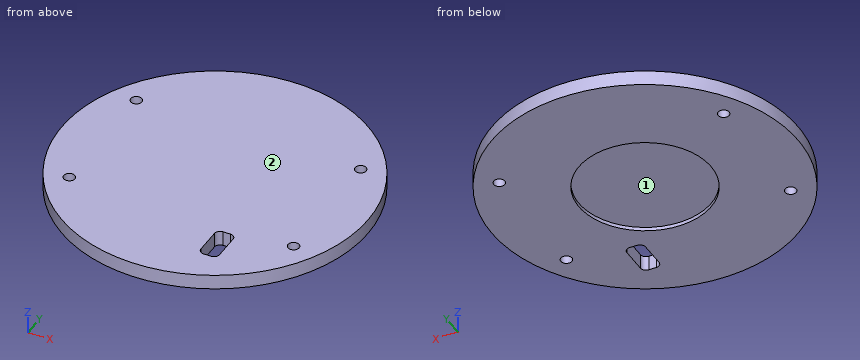
Autodesk Inventor part; units mm, degrees
ref_plane "Work Plane3" through (0, 0, 0) normal (0, 0, 1) x (1, 0, 0)
ref_plane "Work Plane4" through (0, 0, 0) normal (0, 0, 1) x (1, 0, 0)
ref_plane "YZ Plane" through (0, 0, 0) normal (1, 0, 0) x (0, 1, 0)
sketch "Sketch1" plane through (0, 0, 0) normal (0, 0, 1) x (1, 0, 0)
  circle A0 centre (0, 0) radius 41
  circle A1 centre (0, 0) radius 17.705
  circle A2 centre (0, 0) radius 15
  circle A3 centre (0, 15) radius 0.75
  circle A4 centre (-10.6066, 10.6066) radius 0.75
  circle A5 centre (-15, 0) radius 0.75
  circle A6 centre (-10.6066, -10.6066) radius 0.75
  circle A7 centre (0, -15) radius 0.75
  circle A8 centre (10.6066, -10.6066) radius 0.75
  circle A9 centre (15, 0) radius 0.75
  circle A10 centre (10.6066, 10.6066) radius 0.75
  dimension "d4" = 30
  dimension "d0" = 82
  dimension "d3" = 35.41
  dimension "d5" = 1.5
  dimension "d6" = 360
sketch "Sketch2" plane through (0, 0, 0) normal (0, 0, 1) x (1, 0, 0)
  circle A0 centre (-30.094, -17.375) radius 1.5
  circle A1 centre (-30.094, 17.375) radius 1.5
  circle A2 centre (30.094, 17.375) radius 1.5
  circle A3 centre (30.094, -17.375) radius 1.5
  point P0 (0, 0)
  dimension "d7" = 3
  dimension "d8" = 3
  dimension "d9" = 3
  dimension "d10" = 3
  dimension "d11" = 17.375
  dimension "d12" = 30.094
  dimension "d13" = 30.094
  dimension "d14" = 17.375
  dimension "d15" = 17.375
  dimension "d16" = 30.094
  dimension "d17" = 17.375
  dimension "d18" = 30.094
extrude "Extrusion1" add sketch "Sketch1" against normal blind 4 contours A0 | A1 | A2 A9 | A2 A9 | A9 A2 A8 A7 A6 A5 A4 A3 A10 | A10 A2 | A2 A10 | A8 A2 | A2 A8 | A3 A2 | A2 A3 | A7 A2 | A2 A7 | A4 A2 | A2 A4 | A6 A2 | A2 A6 | A5 A2 | A2 A5
extrude "Extrusion2" cut sketch "Sketch2" against normal blind 4
ref_plane "Work Plane1" through (0, 0, -4) normal (0, 0, 1) x (1, 0, 0)
ref_plane "Work Plane2" through (0, 0, -4) normal (0, 0, 1) x (1, 0, 0)
ref_plane "Work Plane3" through (0, 0, 0) normal (0, 0, 1) x (1, 0, 0)
sketch "Sketch5" plane through (0, 0, 0) normal (0, 0, 1) x (1, 0, 0)
  line L0 (11, -30) -> (16, -30)
  line L1 (16, -30) -> (16, -20)
  line L2 (16, -20) -> (11, -20)
  line L3 (11, -20) -> (11, -30)
  point P0 (0, 0)
  point P1 (13.5, -20)
  point P2 (13.5, -30)
  point P3 (16, -25)
  dimension "d44" = 5
  dimension "d45" = 10
  dimension "d54" = 11
  dimension "d55" = 20
extrude "Extrusion5" cut sketch "Sketch5" against normal blind 4
fillet "Fillet1" radius 1.5 4 edges at (11, -20, -2) (11, -30, -2) (16, -20, -2) (16, -30, -2)
ref_plane "Work Plane4" through (0, 0, 0) normal (0, 0, 1) x (1, 0, 0)
ref_plane "Work Plane5" through (0, 0, -4) normal (0, 0, -1) x (-1, 0, 0)
sketch "Sketch7" plane through (0, 0, -4) normal (0, 0, -1) x (-1, 0, 0)
  circle A0 centre (0, 0) radius 17.705
  circle A1 centre (0, 0) radius 15
  circle A2 centre (0, 15) radius 2.5
  circle A3 centre (-10.6066, 10.6066) radius 2.5
  circle A4 centre (-15, 0) radius 2.5
  circle A5 centre (-10.6066, -10.6066) radius 2.5
  circle A6 centre (0, -15) radius 2.5
  circle A7 centre (10.6066, -10.6066) radius 2.5
  circle A8 centre (15, 0) radius 2.5
  circle A9 centre (10.6066, 10.6066) radius 2.5
  circle A10 centre (0, 0) radius 4.25
  circle A11 centre (0, 0) radius 2.5
  point P0 (0, 0)
  point P1 (0, 0)
  point P2 (0, -4)
  point P3 (0, -19)
  dimension "d60" = 35.41
  dimension "d61" = 5
  dimension "d62" = 360
  dimension "d63" = 8.5
  dimension "d64" = 5
  dimension "d65" = 15
  dimension "d66" = 15
extrude "Extrusion6" cut sketch "Sketch7" against normal blind 1 contours A0 | A1 A8 | A1 A8 | A8 A1 A7 A6 A5 A4 A3 A2 A9 | A9 A1 | A1 A9 | A7 A1 | A1 A7 | A2 A1 | A1 A2 | A6 A1 | A1 A6 | A3 A1 | A1 A3 | A5 A1 | A1 A5 | A4 A1 | A1 A4 | A10 | A11
properties part number "lower-plate_3DPrint"
Part model, mm, in its own coordinate system. Face numbers are marked on the shaded views. Give positions to 0.01 mm unless a question says otherwise; leave off trailing zeros. Write each loop counter-clockwise with the first axis right and the second up, starting at its lowest first coordinate (ties: lowest second). Pieces come first, ordered by that corner, then holes. Notation, with made-up numbers: M 21.25,17.5 L 39.25,17.5 A6 ccw 39.25,21.5 Z; hole C -29,-23 d11. An arc over 180 degrees is marked long. Use CSV: the item, a comma, the result in double quotes.
Item 1: Pull direction X, two halves, no side cores. Call the marked faces 1 and 2: +X half, -X half, draft (parallel to the pull), parting line (faces both ways), or undercut.
Taken from the geometry:
face 1,"undercut"
face 2,"draft"
Item 2: Pin check, flat tips, straight feed: P1, Ø3.5, axis at x = 30.094, y = -17.375, coming from the +Z side; P2, Ø1, axis at x = 14, z = -2, coming from the +Y side; P3, Ø1, axis at y = -10, z = -1.5, coming from the +X side; P4, Ø2, axis at y = -24, z = -1.5, coming from the +X side. Stop position of each tip, or through.
Taken from the geometry:
P1,"stops at z = 0"
P2,"stops at y = 38.71"
P3,"stops at x = 39.88"
P4,"stops at x = 33.94"
Item 3: Drill centre lines: probe 1 along Y at (x, z) = (0, -3.65) (3 decimals); probe 2 along Y at (x, z) = (-31, -3); probe 3 along Y at (x, z) = (-16, -3.6). Where is each one in solid material? Low to high.
Taken from the geometry:
probe 1,"y = -41 to -17.705, 17.705 to 41"
probe 2,"y = -26.83 to -18.57, -16.18 to 16.18, 18.57 to 26.83"
probe 3,"y = -37.75 to -7.58, 7.58 to 37.75"
Item 4: Slice it at B-B on y = -24.5. Write the cut outline in (x, z).
Taken from the geometry:
outline,"M -32.87,-4 L 11,-4 L 11,0 L -32.87,0 Z; M 16,-4 L 32.87,-4 L 32.87,0 L 16,0 Z"
Item 5: Slice it at A-A on x = 0. Write the cut outline in (y, z) (3 decimals), plus the area to 3 significant figures.
Taken from the geometry:
outline,"M -41,-4 L -17.705,-4 L -17.705,-3 L 17.705,-3 L 17.705,-4 L 41,-4 L 41,0 L -41,0 Z"
area,"293 mm²"
Item 6: Slice it at D-D on z = -2.2. Write the cut outline in (x, y) (3 decimals).
Taken from the geometry:
outline,"C 0,0 d82; hole C -30.094,-17.375 d3; hole C -30.094,17.375 d3; hole M 11,-28.5 A1.5 ccw 12.5,-30 L 14.5,-30 A1.5 ccw 16,-28.5 L 16,-21.5 A1.5 ccw 14.5,-20 L 12.5,-20 A1.5 ccw 11,-21.5 Z; hole C 30.094,-17.375 d3; hole C 30.094,17.375 d3"
